from build123d import *

# Parameters (mm, degrees)
SKETCH1_R           = 2.1082
SKETCH1_R_2         = 3.475
SKETCH1_W           = 66.2
SKETCH1_H           = 30.2
BOSS_EXTRUDE1_DEPTH = 6.35


with BuildPart() as part:
    # Sketch1 → Boss-Extrude1 (new body)
    with BuildSketch(Plane(origin=(0, 0, 0), x_dir=(1, 0, 0), z_dir=(0, 1, 0))):
        Polygon((59.986534985, 21.9), (-17.836534985, 21.9), (-23.836534985, 15.9), (-23.836534985, -15.1), (-17.836534985, -21.1), (-5.201359875, -21.1), (2.025, -28.326359875), (2.025, -31.939539813), (5.638179938, -35.55271975), (35.711820062, -35.55271975), (39.325, -31.939539813), (39.325, -28.326359875), (46.551359875, -21.1), (59.986534985, -21.1), (65.986534985, -15.1), (65.986534985, 15.9), align=None)
        with Locations(Location((58.675, 9.25, 0), (0, 0, 270))):
            Circle(SKETCH1_R, mode=Mode.SUBTRACT)
        with Locations(Location((58.675, -9.25, 0), (0, 0, 90))):
            Circle(SKETCH1_R, mode=Mode.SUBTRACT)
        with Locations(Location((-16.525, -9.25, 0), (0, 0, 270))):
            Circle(SKETCH1_R, mode=Mode.SUBTRACT)
        with Locations(Location((-16.525, 9.25, 0), (0, 0, 90))):
            Circle(SKETCH1_R, mode=Mode.SUBTRACT)
        with Locations(Location((11.15, -26.022, 0), (0, 0, 270))):
            Circle(SKETCH1_R_2, mode=Mode.SUBTRACT)
        with Locations(Location((30.2, -26.022, 0), (0, 0, 90))):
            Circle(SKETCH1_R_2, mode=Mode.SUBTRACT)
        with Locations((21.075, 0)):
            Rectangle(SKETCH1_W, SKETCH1_H, mode=Mode.SUBTRACT)
    extrude(amount=BOSS_EXTRUDE1_DEPTH)


solid = part.part
Input: part model. Units: mm. Frame: model coordinates. A direction names the side the tool comes from. Round coordinates to 2 decimals unless told otherwise and drop trailing zeros. Loops run counter-clockwise (first coordinate to the right, second up) from the corner with the lowest first, then second, coordinate; pieces in that order, holes last. Notation, with made-up numbers: M -25.75,-25 L -4.75,-25 A21 cw -4.75,1 Z; hole C 55.25,55.5 d5. An arc over 180 degrees is marked long. Answer as CSV lines item,"result". Start each with the question number.
(1) Section D-D, the plane x = 50. Output: boundary loops of the cut face in (y, z).
(2) Line query: line 1 (Z direction, x = 58.5, y = 1.25); line 2 (X direction, y = 1.25, z = 9) (3 decimals); line 3 (Z direction, x = 30.2, y = 3.5). Output: solid intervals per line, ascending. Write a range as [from, to].
(3) Draft query along X for faces 4 (the cylindrical face through (-18.615, 3.131, -8.976)), 5 (the flat face through (42.89, 3.13, 24.76)), 6 (the flat face through (-20.879, 3.131, 18.058)). Return one class per face: released by +X, released by -X, zero draft, split by the parting line, or undercut.
(4) Section B-B, the plane x = 30.2. Output: boundary loops of the cut face in (y, z).
(5) Section A-A, the plane z = 9.25. Output: boundary loops of the cut face in (x, y) (3 decimals), plus the area to 3 significant figures.
(6) Section C-C, the plane z = -3. Output: boundary loops of the cut face in (x, y) (3 decimals).
(7) First-contact query: pin 1 (1.1 mm diameter, centred on y = 2, z = 31, fed in from +X) (3 decimals). Flat tip, straight axial feed; report the tip coordinate or a pass-through.
(8) Reachability of faces 1 (the flat face through (39.325, 3, 30)), 2 (the flat face through (2.025, 3, 30)), 3 (the flat face through (21, 3, -15.1)) from +Z, -Z, +X, -X, +Y, -Y: full face, straight path, thin tool, end or side. Return the list, or none.
Values found:
1,outline,"M 0,-21.9 L 6.35,-21.9 L 6.35,-15.1 L 0,-15.1 Z; M 0,15.1 L 6.35,15.1 L 6.35,21.1 L 0,21.1 Z"
2,line 1,"z = [-21.9, -11.35], [-7.15, 7.15], [11.35, 21.1]"
2,line 2,"x = [-23.837, -18.618], [-14.432, -12.025], [54.175, 56.582], [60.768, 65.987]"
2,line 3,"z = [-21.9, -15.1], [15.1, 22.55], [29.5, 35.55]"
3,face 4,"undercut"
3,face 5,"released by +X"
3,face 6,"released by -X"
4,outline,"M 0,-21.9 L 6.35,-21.9 L 6.35,-15.1 L 0,-15.1 Z; M 0,15.1 L 6.35,15.1 L 6.35,22.55 L 0,22.55 Z; M 0,29.5 L 6.35,29.5 L 6.35,35.55 L 0,35.55 Z"
5,outline,"M -23.837,0 L -18.633,0 L -18.633,6.35 L -23.837,6.35 Z; M -14.417,0 L -12.025,0 L -12.025,6.35 L -14.417,6.35 Z; M 54.175,0 L 56.567,0 L 56.567,6.35 L 54.175,6.35 Z; M 60.783,0 L 65.987,0 L 65.987,6.35 L 60.783,6.35 Z"
5,area,"96.5 mm²"
6,outline,"M -23.837,0 L -12.025,0 L -12.025,6.35 L -23.837,6.35 Z; M 54.175,0 L 65.987,0 L 65.987,6.35 L 54.175,6.35 Z"
7,pin 1,"stops at x = 39.325"
8,face 1,"+Z, +X, +Y, -Y"
8,face 2,"+Z, -X, +Y, -Y"
8,face 3,"+Y, -Y"
